Design review of the part built by this model. Coordinates are the model's own, in mm. Give positions to 0.01 mm unless a question says otherwise; leave off trailing zeros. Write each loop counter-clockwise with the first axis right and the second up, starting at its lowest first coordinate (ties: lowest second). Pieces come first, ordered by that corner, then holes. Notation, with made-up numbers: M 55,44.5 L 101,44.5 A24 cw 101,66.5 Z; hole C 57,3 d8. An arc over 180 degrees is marked long. Use a Markdown table: item, result. Add a question column.
```python
from build123d import *

# Parameters (mm, degrees)
ESQUISSE1_R              = 7.5
ESQUISSE1_R_2            = 2.3
BOSS_EXTRU_1_DEPTH       = 6
ENL_V_MAT_EXTRU_9_DEPTH  = 10.5
ESQUISSE6_R              = 2.3
ENL_V_MAT_EXTRU_10_DEPTH = 50
ENL_V_MAT_EXTRU_11_DEPTH = 50
ESQUISSE9_R              = 2.5
ENL_V_MAT_EXTRU_12_DEPTH = 35
ESQUISSE11_R             = 2.3
ENL_V_MAT_EXTRU_15_DEPTH = 10


with BuildPart() as part:
    # Esquisse1 → Boss.-Extru.1 (new body)
    with BuildSketch(Plane(origin=(0, 0, 0), x_dir=(1, 0, 0), z_dir=(0, 1, 0))):
        Polygon((-150, 0), (-150, 260), (-110, 300), (110, 300), (150, 260), (150, 0), align=None)
        with Locations(Location((-120, 30, 0), (0, 0, 270))):
            Circle(ESQUISSE1_R, mode=Mode.SUBTRACT)
        with Locations(Location((-120, 267.5, 0), (0, 0, 270))):
            Circle(ESQUISSE1_R, mode=Mode.SUBTRACT)
        with Locations(Location((120, 267.5, 0), (0, 0, 270))):
            Circle(ESQUISSE1_R, mode=Mode.SUBTRACT)
        with Locations(Location((-111.514718626, 275.985281374, 0), (0, 0, 270))):
            Circle(ESQUISSE1_R_2, mode=Mode.SUBTRACT)
        with Locations(Location((-128.485281374, 259.014718626, 0), (0, 0, 270))):
            Circle(ESQUISSE1_R_2, mode=Mode.SUBTRACT)
        with Locations(Location((111.514718626, 275.985281374, 0), (0, 0, 270))):
            Circle(ESQUISSE1_R_2, mode=Mode.SUBTRACT)
        with Locations(Location((128.485281374, 259.014718626, 0), (0, 0, 270))):
            Circle(ESQUISSE1_R_2, mode=Mode.SUBTRACT)
        with Locations(Location((120, 30, 0), (0, 0, 270))):
            Circle(ESQUISSE1_R, mode=Mode.SUBTRACT)
        with Locations(Location((120, 42, 0), (0, 0, 270))):
            Circle(ESQUISSE1_R_2, mode=Mode.SUBTRACT)
        with Locations(Location((-120, 42, 0), (0, 0, 270))):
            Circle(ESQUISSE1_R_2, mode=Mode.SUBTRACT)
        with Locations(Location((-120, 18, 0), (0, 0, 270))):
            Circle(ESQUISSE1_R_2, mode=Mode.SUBTRACT)
        with Locations(Location((-132, 30, 0), (0, 0, 270))):
            Circle(ESQUISSE1_R_2, mode=Mode.SUBTRACT)
        with Locations(Location((-108, 30, 0), (0, 0, 270))):
            Circle(ESQUISSE1_R_2, mode=Mode.SUBTRACT)
        with Locations(Location((108, 30, 0), (0, 0, 270))):
            Circle(ESQUISSE1_R_2, mode=Mode.SUBTRACT)
        with Locations(Location((132, 30, 0), (0, 0, 270))):
            Circle(ESQUISSE1_R_2, mode=Mode.SUBTRACT)
        with Locations(Location((120, 18, 0), (0, 0, 270))):
            Circle(ESQUISSE1_R_2, mode=Mode.SUBTRACT)
    extrude(amount=BOSS_EXTRU_1_DEPTH)

    # Esquisse7 → Enlèv. mat.-Extru.9 (cut)
    with BuildSketch(Plane(origin=(0, 6, 0), x_dir=(1, 0, 0), z_dir=(0, 1, 0))):
        Polygon((-130, 150), (-130, 182), (-140, 182), (-140, 118), (-130, 118), align=None)
    enl_v_mat_extru_9 = extrude(amount=-ENL_V_MAT_EXTRU_9_DEPTH, mode=Mode.SUBTRACT)

    # Esquisse6 → Enlèv. mat.-Extru.10 (cut)
    with BuildSketch(Plane(origin=(0, 6, 0), x_dir=(1, 0, 0), z_dir=(0, 1, 0))):
        with Locations(Location((-138.5, 90, 0), (0, 0, 270))):
            Circle(ESQUISSE6_R)
        with Locations(Location((-138.5, 112, 0), (0, 0, 270))):
            Circle(ESQUISSE6_R)
        with Locations(Location((-106.5, 112, 0), (0, 0, 270))):
            Circle(ESQUISSE6_R)
        with Locations(Location((-106.5, 90, 0), (0, 0, 270))):
            Circle(ESQUISSE6_R)
    enl_v_mat_extru_10 = extrude(amount=-ENL_V_MAT_EXTRU_10_DEPTH, mode=Mode.SUBTRACT)

    # Esquisse4 → Enlèv. mat.-Extru.11 (cut)
    with BuildSketch(Plane(origin=(0, 6, 0), x_dir=(1, 0, 0), z_dir=(0, 1, 0))):
        Polygon((-100, 150), (-100, 182), (-64, 182), (-64, 118), (-100, 118), align=None)
    enl_v_mat_extru_11 = extrude(amount=-ENL_V_MAT_EXTRU_11_DEPTH, mode=Mode.SUBTRACT)

    # Symétrie1: Enlèv. mat.-Extru.9 across plane
    add(enl_v_mat_extru_9.mirror(Plane(origin=(0, 0, 0), x_dir=(0, 0, 1), z_dir=(1, 0, 0))), mode=Mode.SUBTRACT)

    # Symétrie2: Enlèv. mat.-Extru.11 across plane
    add(enl_v_mat_extru_11.mirror(Plane(origin=(0, 0, 0), x_dir=(0, 0, 1), z_dir=(1, 0, 0))), mode=Mode.SUBTRACT)

    # Symétrie3: Enlèv. mat.-Extru.10 across plane
    add(enl_v_mat_extru_10.mirror(Plane(origin=(0, 0, 0), x_dir=(0, 0, 1), z_dir=(1, 0, 0))), mode=Mode.SUBTRACT)

    # Esquisse9 → Enlèv. mat.-Extru.12 (cut)
    with BuildSketch(Plane(origin=(0, 6, 0), x_dir=(1, 0, 0), z_dir=(0, 1, 0))):
        with Locations(Location((-100, 50, 0), (0, 0, 270))):
            Circle(ESQUISSE9_R)
        with Locations(Location((100, 50, 0), (0, 0, 270))):
            Circle(ESQUISSE9_R)
        with Locations(Location((100, 250, 0), (0, 0, 270))):
            Circle(ESQUISSE9_R)
        with Locations(Location((-100, 250, 0), (0, 0, 270))):
            Circle(ESQUISSE9_R)
    extrude(amount=-ENL_V_MAT_EXTRU_12_DEPTH, mode=Mode.SUBTRACT)

    # Esquisse11 → Enlèv. mat.-Extru.15 (cut)
    with BuildSketch(Plane(origin=(0, 6, 0), x_dir=(1, 0, 0), z_dir=(0, 1, 0))):
        with Locations(Location((36, 116, 0), (0, 0, 270))):
            Circle(ESQUISSE11_R)
        with Locations(Location((60, 116, 0), (0, 0, 270))):
            Circle(ESQUISSE11_R)
        with Locations(Location((60, 174, 0), (0, 0, 270))):
            Circle(ESQUISSE11_R)
        with Locations(Location((-19, 227, 0), (0, 0, 270))):
            Circle(ESQUISSE11_R)
        with Locations(Location((-19, 183, 0), (0, 0, 270))):
            Circle(ESQUISSE11_R)
        with Locations(Location((33, 227, 0), (0, 0, 270))):
            Circle(ESQUISSE11_R)
        with Locations(Location((19, 117, 0), (0, 0, 270))):
            Circle(ESQUISSE11_R)
        with Locations(Location((19, 73, 0), (0, 0, 270))):
            Circle(ESQUISSE11_R)
        with Locations(Location((-33, 73, 0), (0, 0, 270))):
            Circle(ESQUISSE11_R)
        with Locations(Location((-60, 126, 0), (0, 0, 270))):
            Circle(ESQUISSE11_R)
        with Locations(Location((-36, 184, 0), (0, 0, 270))):
            Circle(ESQUISSE11_R)
        with Locations(Location((-60, 184, 0), (0, 0, 270))):
            Circle(ESQUISSE11_R)
    extrude(amount=-ENL_V_MAT_EXTRU_15_DEPTH, mode=Mode.SUBTRACT)


solid = part.part
```
(1) Add section B-B on y = 2.6. Give the number of separate pieces and of enclosed holes in the cut face, then the cut area to 3 significant figures.
(2) Wall thickness on L1, parallel to X at y = 2.1, z = -90; L2, parallel to X at y = 4.35, z = -227; L3, parallel to X at y = 1.5, z = -50: over which ranges is each line inside the solid? List them lowest first.
(3) The part is to be moulded in two halves that separate along X. For faces 1 (the flat face through (2, 6, -152)), 2 (the cylindrical face through (-122.87, 2.96, -260.57)), 3 (the flat face through (-130, 3, -280)), say which applies: released by +X, released by -X, zero draft, split by the parting line, or undercut.
(4) Add section A-A on z = -135. Give the boundary of the cut face in (x, y), then the cut area to 3 significant figures.
From the geometry:
| question | item | result |
|---|---|---|
| 1 | separate pieces | 1 |
| 1 | enclosed holes | 44 |
| 1 | area | 81,200 mm^2 |
| 2 | L1 | x = -150 to -140.8, -136.2 to -108.8, -104.2 to 104.2, 108.8 to 136.2, 140.8 to 150 |
| 2 | L2 | x = -150 to -21.3, -16.7 to 30.7, 35.3 to 150 |
| 2 | L3 | x = -150 to -102.5, -97.5 to 97.5, 102.5 to 150 |
| 3 | face 1 | zero draft |
| 3 | face 2 | undercut |
| 3 | face 3 | released by -X |
| 4 | outline | M -150,0 L -140,0 L -140,6 L -150,6 Z; M -130,0 L -100,0 L -100,6 L -130,6 Z; M -64,0 L 64,0 L 64,6 L -64,6 Z; M 100,0 L 130,0 L 130,6 L 100,6 Z; M 140,0 L 150,0 L 150,6 L 140,6 Z |
| 4 | area | 1,250 mm^2 |
